Part model, mm, in its own coordinate system. A direction names the side the tool comes from. Round coordinates to 2 decimals unless told otherwise and drop trailing zeros. Loops run counter-clockwise (first coordinate to the right, second up) from the corner with the lowest first, then second, coordinate; pieces in that order, holes last. Notation, with made-up numbers: M 64.25,57 L 89.25,57 A19 cw 89.25,82 Z; hole C 54,-34.5 d2. An arc over 180 degrees is marked long. Write each question's results on one line, items separated by ' | '.
from build123d import *

# Parameters (mm, degrees)
F0_R     = 18.542
F0_R_2   = 1.7526
F1_DEPTH = 9.525


with BuildPart() as f1:
    # F0 (on Top) → F1 (new body)
    with BuildSketch(Plane.XY):
        Circle(F0_R)
        with BuildLine():
            ThreePointArc((-5.031432, -4.737986), (-5.98522, -3.455569), (-6.618932, -1.988355))
            Line((-6.618932, -1.988355), (-9.781322, -2.93835))
            ThreePointArc((-9.781322, -2.93835), (-8.844836, 5.106569), (-2.345975, 9.940049))
            Line((-2.345975, 9.940049), (-1.5875, 6.726341))
            ThreePointArc((-1.5875, 6.726341), (0, 6.911137), (1.5875, 6.726341))
            Line((1.5875, 6.726341), (2.345975, 9.940049))
            ThreePointArc((2.345975, 9.940049), (8.844836, 5.106569), (9.781322, -2.93835))
            Line((9.781322, -2.93835), (6.618932, -1.988355))
            ThreePointArc((6.618932, -1.988355), (5.98522, -3.455569), (5.031432, -4.737986))
            Line((5.031432, -4.737986), (7.435347, -7.001698))
            ThreePointArc((7.435347, -7.001698), (0, -10.213137), (-7.435347, -7.001698))
            Line((-7.435347, -7.001698), (-5.031432, -4.737986))
        make_face(mode=Mode.SUBTRACT)
        with Locations((-13.716, 0)):
            Circle(F0_R_2, mode=Mode.SUBTRACT)
        with Locations((13.716, 0)):
            Circle(F0_R_2, mode=Mode.SUBTRACT)
    extrude(amount=F1_DEPTH)


solid = f1.part
Item 1: Band-saw the part on C-C on z = 8.25. Give the cut face in (x, y).
Filled sheet:
outline: C 0,0 d37.08; hole C -13.72,0 d3.51; hole M -9.78,-2.94 L -6.62,-1.99 A6.91 ccw -5.03,-4.74 L -7.44,-7 A10.21 ccw 7.44,-7 L 5.03,-4.74 A6.91 ccw 6.62,-1.99 L 9.78,-2.94 A10.21 ccw 2.35,9.94 L 1.59,6.73 A6.91 ccw -1.59,6.73 L -2.35,9.94 A10.21 ccw Z; hole C 13.72,0 d3.51
Item 2: Band-saw the part on B-B on y = 0. Give the cut face in (x, z) (3 decimals), and give its area (3 significant figures).
Filled sheet:
outline: M -18.542,0 L -15.469,0 L -15.469,9.525 L -18.542,9.525 Z; M -11.963,0 L -10.213,0 L -10.213,9.525 L -11.963,9.525 Z; M 10.213,0 L 11.963,0 L 11.963,9.525 L 10.213,9.525 Z; M 15.469,0 L 18.542,0 L 18.542,9.525 L 15.469,9.525 Z | area: 91.9 mm^2
Item 3: Drop flat-ended pins along their axis: P1, Ø1.5, axis at y = -12, z = 1.5, coming from the +X side; P2, Ø1.5, axis at x = 13.5, z = 4, coming from the +Y side; P3, Ø5, axis at x = 5.5, z = 4.5, coming from the -Y side; P4, Ø2, axis at x = -13.716, y = 0, coming from the +Z side. Give the stop position or say it passes through.
Filled sheet:
P1: x = 14.74 | P2: y = 13.46 | P3: y = -18.3 | P4: through
Item 4: Wall check: L1, parallel to Y at x = -4, z = 8; L2, parallel to X at y = 8, z = 5.25; L3, parallel to Y at x = 3, z = 2.75. Give the ranges that are in metal, low to high.
Filled sheet:
L1: -18.11 to -9.4, 9.4 to 18.11 | L2: -16.73 to -6.35, -1.89 to 1.89, 6.35 to 16.73 | L3: -18.3 to -9.76, 9.76 to 18.3
Item 5: Band-saw the part on A-A on x = 0. Give the cut face in (y, z) (3 decimals).
Filled sheet:
outline: M -18.542,0 L -10.213,0 L -10.213,9.525 L -18.542,9.525 Z; M 6.911,0 L 18.542,0 L 18.542,9.525 L 6.911,9.525 Z
Item 6: Band-saw the part on D-D on x = -14. Give the cut face in (y, z) (3 decimals), and give its area (3 significant figures).
Filled sheet:
outline: M -12.158,0 L -1.729,0 L -1.729,9.525 L -12.158,9.525 Z; M 1.729,0 L 12.158,0 L 12.158,9.525 L 1.729,9.525 Z | area: 199 mm^2
Item 7: Which spindle directions (+Z, -Z, +X, -X, +Y, -Y) get a long thin tool onto all of the face, cutting with end or side? Do faces 4 (the flat face through (8, -4, 9.525)), 5 (the flat face through (-1.972, 8.356, 4.696)). Say none if no direction does.
Filled sheet:
face 4: +Z, +X, -X, +Y, -Y | face 5: +Z, -Z
Item 8: Two-plate mould, pull along X, no slides. Class faces 1 (the cylindrical face through (-13.67, 12.53, 4.7)), 2 (the cylindrical face through (-8.9, 5.01, 4.7)), 3 (the flat face through (8, -4, 0)): +X half, -X half, draft (parallel to the pull), parting line (faces both ways), or undercut.
Filled sheet:
face 1: parting line | face 2: undercut | face 3: draft
